Autodesk Fusion 360 part; units mm, degrees
sketch "Sketch2" plane through (0, 0, 0) normal (0, 1, 0) x (1, 0, 0)
  line L0 (0, 4) -> (18.2, 4)
  line L1 (18.2, 4) -> (18.2, -4)
  line L2 (18.2, -4) -> (0, -4)
  line L3 (0, -4) -> (0, 4)
  line L4 (8.4, 4) -> (8.4, -4)
  line L5 (0, 0) -> (8.4, 0) construction
  line L6 (4.2, 4) -> (4.2, -4) construction
  line L7 (0, 4) -> (-4, 4)
  line L8 (-4, 4) -> (-4, -4)
  line L9 (-4, -4) -> (0, -4)
  line L10 (0, -4) -> (0, 4)
  point P0 (4.2, 0)
  dimension "d5" = 8
  dimension "d6" = 8.4
  dimension "d7" = 14
  dimension "d14" = 4
  dimension "d15" = 9.8
extrude "Extrude2" add sketch "Sketch2" along normal blind 8 contours L0 L2 L3 L4 L10
extrude "Extrude3" add sketch "Sketch2" against normal blind 4.2
chamfer "Chamfer1" distance 1 angle 45 2 edges at (0, 8, 0) (8.4, 8, 0)
sketch "Sketch1" plane through (0, 0, 0) normal (0, 1, 0) x (1, 0, 0)
  line L0 (3, -2.5) -> (-3, -2.5)
  line L1 (-3, -2.5) -> (-3, 2.5)
  line L2 (-3, 2.5) -> (3, 2.5)
  line L3 (3, 2.5) -> (3, -2.5)
  line L4 (3, -2.5) -> (-3, 2.5) construction
  line L5 (-3, -2.5) -> (3, 2.5) construction
  dimension "d1" = 5
  dimension "d2" = 6
extrude "Extrude1" [suppressed]
The model under review builds one solid part; all positions refer to its coordinate system, in mm. A direction names the side the tool comes from. Round coordinates to 2 decimals unless told otherwise and drop trailing zeros. Order: outer loops, then holes, each group sorted by start corner. A loop starts at its lowest first (then second) coordinate and runs counter-clockwise, first axis right, second up. Notation, with made-up numbers: (59.5, 86.5) - (107.5, 86.5) arc R25 ccw to (107.5, 110.5) - close; hole circle Ø4 at (15, 86). An arc over 180 degrees is marked (long way). Answer in a Markdown table with one row per item.
(1) Take a section at A-A on z = 2.75. Write out the cut boundary in (x, y), plus the area to 3 significant figures.
Result set:
| item | result |
|---|---|
| outline | (-4, -4.2) - (18.2, -4.2) - (18.2, 0) - (8.4, 0) - (8.4, 7) - (7.4, 8) - (1, 8) - (0, 7) - (0, 0) - (-4, 0) - close |
| area | 159 mm2 |
(2) Clearance check with flat-ended pins moving along their axes: P1, Ø2, axis at y = 4.5, z = -1, coming from the +X side; P2, Ø1.5, axis at y = 5, z = 0, coming from the -X side; P3, Ø2, axis at x = -2.5, z = -1, coming from the +Y side. State where each tip first meets the part, or that it passes through.
Result set:
| item | result |
|---|---|
| P1 | stops at x = 8.4 |
| P2 | stops at x = 0 |
| P3 | stops at y = 0 |
(3) Take a section at C-C on x = 10.25. Write out the cut boundary in (y, z), plus the area to 3 significant figures.
Result set:
| item | result |
|---|---|
| outline | (-4.2, -4) - (0, -4) - (0, 4) - (-4.2, 4) - close |
| area | 33.6 mm2 |
(4) Machinability: for faces 1 (the face through (-2, 0, 0)), 2 (the face through (-4, -2, 0)), 3 (the face through (8.4, 3, 0)), which of the approach directions +Z, -Z, +X, -X, +Y, -Y give a long, thin tool a straight path to every point of the face, cutting with its end or side? Answer none if there is none.
Result set:
| item | result |
|---|---|
| face 1 | +Z, -Z, -X, +Y |
| face 2 | +Z, -Z, -X, +Y, -Y |
| face 3 | +Z, -Z, +X, +Y |
(5) Take a section at B-B on y = 3. Write out the cut boundary in (x, z).
Result set:
| item | result |
|---|---|
| outline | (0, -4) - (8.4, -4) - (8.4, 4) - (0, 4) - close |
(6) For line 1 (Y direction, x = -2, z = 3.25); line 2 (X direction, y = 6, z = 3.75); line 3 (Y direction, x = 0.5, z = -2.25), list the stretches that pass through material, from the lowest coordinate up. Write a range as from..to.
Result set:
| item | result |
|---|---|
| line 1 | y = -4.2..0 |
| line 2 | x = 0..8.4 |
| line 3 | y = -4.2..7.5 |
